The listing builds one solid part. Answer for the finished solid, in the listing's coordinates (mm). Face numbers are marked on the shaded views. Round coordinates to 2 decimals unless told otherwise and drop trailing zeros. Write each loop counter-clockwise with the first axis right and the second up, starting at its lowest first coordinate (ties: lowest second). Pieces come first, ordered by that corner, then holes. Notation, with made-up numbers: (-20, -2) - (24, -2) arc R8 ccw to (24, 8) - close; hole circle Ø5 at (40, 59.25). An arc over 180 degrees is marked (long way). Return JSON: item names as keys, results as strings. Group by question number.
(1) Find the intervals of material crossed by line 1 along Z through (x, y) = (115, 3); line 2 along Y through (x, z) = (117.5, -21); line 3 along Z through (x, y) = (40, 34.5), in increasing order. Write a range as [from, to].
(2) Section A-A, the plane x = 120.5 is taken. Write down the section's boundary in (y, z), then the cut area to 3 significant figures.
(3) Section B-B, the plane x = 165 is taken. Write down the section's boundary in (y, z), then the cut area to 3 significant figures.
(4) Determine the mould class of the marked faces 1, 2, 3 and 4 for opening direction Y: +Y half, -Y half, draft (parallel to the pull), parting line (faces both ways), or undercut.
(5) Each of these flat-tipped pins is pushed along its axis until it touches: pin 1 (8 mm diameter, centred on x = 156, z = -41.5, fed in from +Y); pin 2 (2.5 mm diameter, centred on y = -3, z = 50, fed in from -X); pin 3 (5.5 mm diameter, centred on x = 137.5, y = 35, fed in from -Z); pin 4 (12 mm diameter, centred on y = 22, z = 24.5, fed in from +X). Where does it stop, or does it pass through?
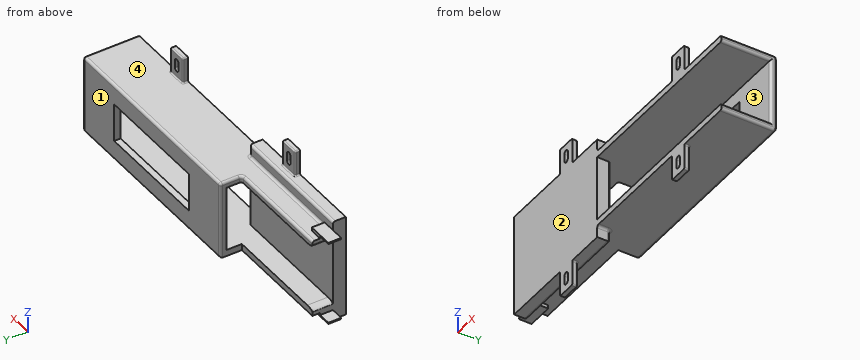
```python
from build123d import *

# Parameters (mm, degrees)
SKETCH1_W                 = 100
SKETCH1_H                 = 80
BOSS_EXTRUDE1_DEPTH       = 5
BOSS_EXTRUDE2_DEPTH       = 15
BOSS_EXTRUDE4_DEPTH       = 150
SKETCH9_W                 = 85
SKETCH9_H                 = 5
BOSS_EXTRUDE5_DEPTH       = 16
SKETCH3_W                 = 15
SKETCH3_H                 = 20
BOSS_EXTRUDE3_DEPTH       = 4
F_4_0MM_START             = -5
F_4_0MM_DOWEL_SLOT1_DEPTH = 4
SKETCH12_W                = 2.75
SKETCH12_H                = 10
BOSS_EXTRUDE7_DEPTH       = 10
SKETCH13_W                = 1
SKETCH13_H                = 10
BOSS_EXTRUDE8_DEPTH       = 10
SKETCH14_W                = 90
SKETCH14_H                = 30
CUT_EXTRUDE1_DEPTH        = 214.187710715
FILLET2_R                 = 2
FILLET3_R                 = 1
FILLET4_SIZE              = 2
FILLET4_SIZE_2            = 6


# Read off the part's stored shape, not the designer's step: Ø4.0mm Dowel Slot1
with BuildPart() as part:
    # Sketch1 → Boss-Extrude1 (new, symmetric)
    with BuildSketch(Plane(origin=(0, 0, 0), x_dir=(1, 0, 0), z_dir=(0, 1, 0))):
        Rectangle(SKETCH1_W, SKETCH1_H)
    extrude(amount=BOSS_EXTRUDE1_DEPTH, both=True)

    # Sketch2 → Boss-Extrude2 (add)
    with BuildSketch(Plane(origin=(50, 0, 0), x_dir=(0, 0, -1), z_dir=(1, 0, 0))):
        Polygon((-30.5, 5), (-30.5, 38), (30.5, 38), (30.5, 5), (25.5, 5), (25.5, 33), (-25.5, 33), (-25.5, 5), align=None)
    extrude(amount=-BOSS_EXTRUDE2_DEPTH)

    # Sketch4 → Boss-Extrude4 (add)
    with BuildSketch(Plane(origin=(50, 0, 0), x_dir=(0, 0, -1), z_dir=(1, 0, 0))):
        Polygon((-30.5, 38), (30.5, 38), (30.5, -5), (25.5, -5), (25.5, 33), (-25.5, 33), (-25.5, -5), (-30.5, -5), align=None)
    extrude(amount=BOSS_EXTRUDE4_DEPTH)

    # Sketch9 → Boss-Extrude5 (add)
    with BuildSketch(Plane(origin=(0, 5, 0), x_dir=(1, 0, 0), z_dir=(0, 1, 0))):
        with Locations((-7.5, -28)):
            Rectangle(SKETCH9_W, SKETCH9_H)
        with Locations((-7.5, 28)):
            Rectangle(SKETCH9_W, SKETCH9_H)
    extrude(amount=BOSS_EXTRUDE5_DEPTH)

    # Sketch3 → Boss-Extrude3 (add)
    with BuildSketch(Plane.XZ.offset(5)):
        with Locations((12.5, 50)):
            Rectangle(SKETCH3_W, SKETCH3_H)
        with Locations((147.5, 40.5)):
            Rectangle(SKETCH3_W, SKETCH3_H)
        with Locations((147.5, -40.5)):
            Rectangle(SKETCH3_W, SKETCH3_H)
        with Locations((12.5, -50)):
            Rectangle(SKETCH3_W, SKETCH3_H)
    extrude(amount=-BOSS_EXTRUDE3_DEPTH)

    # Ø4.0mm Dowel Slot1 outline → Ø4.0mm Dowel Slot1 (cut)
    with BuildSketch(Plane(origin=(0, 0, 0), x_dir=(1, 0, 0), z_dir=(0, 1, 0)).offset(F_4_0MM_START)):
        with BuildLine():
            Line((149.5, 37.5), (149.5, 43.5))
            ThreePointArc((149.5, 43.5), (147.5, 45.5), (145.5, 43.5))
            Line((145.5, 43.5), (145.5, 37.5))
            ThreePointArc((145.5, 37.5), (147.5, 35.5), (149.5, 37.5))
        make_face()
        with BuildLine():
            ThreePointArc((149.5, -37.5), (147.5, -35.5), (145.5, -37.5))
            Line((145.5, -37.5), (145.5, -43.5))
            ThreePointArc((145.5, -43.5), (147.5, -45.5), (149.5, -43.5))
            Line((149.5, -43.5), (149.5, -37.5))
        make_face()
        with BuildLine():
            Line((14.5, -53), (14.5, -47))
            ThreePointArc((14.5, -47), (12.5, -45), (10.5, -47))
            Line((10.5, -47), (10.5, -53))
            ThreePointArc((10.5, -53), (12.5, -55), (14.5, -53))
        make_face()
        with BuildLine():
            ThreePointArc((14.5, 53), (12.5, 55), (10.5, 53))
            Line((10.5, 53), (10.5, 47))
            ThreePointArc((10.5, 47), (12.5, 45), (14.5, 47))
            Line((14.5, 47), (14.5, 53))
        make_face()
    extrude(amount=F_4_0MM_DOWEL_SLOT1_DEPTH, mode=Mode.SUBTRACT)

    # Sketch12 → Boss-Extrude7 (add)
    with BuildSketch(Plane.ZY.offset(50)):
        with Locations((-31.875, 10)):
            Rectangle(SKETCH12_W, SKETCH12_H)
        with Locations((31.875, 10)):
            Rectangle(SKETCH12_W, SKETCH12_H)
    extrude(amount=-BOSS_EXTRUDE7_DEPTH)

    # Sketch13 → Boss-Extrude8 (add)
    with BuildSketch(Plane.ZY.offset(50)):
        with Locations((32.75, 10)):
            Rectangle(SKETCH13_W, SKETCH13_H)
        with Locations((-32.75, 10)):
            Rectangle(SKETCH13_W, SKETCH13_H)
    extrude(amount=BOSS_EXTRUDE8_DEPTH)

    # Sketch14 → Cut-Extrude1 (cut, through all)
    with BuildSketch(Plane(origin=(0, 38, 0), x_dir=(1, 0, 0), z_dir=(0, 1, 0))):
        with Locations((117.5, 0)):
            Rectangle(SKETCH14_W, SKETCH14_H)
    extrude(amount=-CUT_EXTRUDE1_DEPTH, mode=Mode.SUBTRACT)

    # Fillet2
    fillet2_edges = [part.edges().sort_by_distance(p)[0] for p in [
        (0, 5, 40),
        (50, 5, -35.25),
        (5, 5, -30.5),
        (5, 5, 30.5),
        (35, 29.5, 30.5),
        (35, 38, 0),
        (117.5, 38, 30.5),
        (117.5, 38, -30.5),
        (50, 0, 30.5),
        (50, 0, -30.5),
        (50, 5, 35.25),
        (200, 16.5, 30.5),
        (200, 14, 25.5),
        (200, 33, 0),
        (200, 14, -25.5),
        (200, 16.5, -30.5),
        (200, 38, 0),
        (35, 21, 28),
        (-7.5, 21, 30.5),
        (0, 5, -40),
    ]]
    fillet(fillet2_edges, radius=FILLET2_R)

    # Fillet3
    fillet3_edges = [part.edges().sort_by_distance(p)[0] for p in [
        (20, -1, 50),
        (20, -3, 60),
        (12.5, -1, 40),
        (20, -3, 40),
        (5, -1, 50),
        (5, -3, 40),
        (12.5, -1, 60),
        (5, -3, 60),
        (140, -1, 40.5),
        (140, -3, 30.5),
        (147.5, -1, 50.5),
        (140, -3, 50.5),
        (155, -1, 40.5),
        (155, -3, 50.5),
        (147.5, -1, 30.5),
        (155, -3, 30.5),
        (147.5, -1, -30.5),
        (140, -3, -30.5),
        (155, -1, -40.5),
        (155, -3, -30.5),
        (147.5, -1, -50.5),
        (155, -3, -50.5),
        (140, -1, -40.5),
        (140, -3, -50.5),
        (12.5, -1, -40),
        (5, -3, -40),
        (20, -1, -50),
        (20, -3, -40),
        (12.5, -1, -60),
        (20, -3, -60),
        (5, -1, -50),
        (5, -3, -60),
        (50, 5, 0),
    ]]
    fillet(fillet3_edges, radius=FILLET3_R)

    # Fillet4
    # an asymmetric fillet: 6, 2 mm, written as the material it takes off along each edge
    with BuildSketch(Plane(origin=(-50, 5, 25.5), x_dir=(0, 0, 1), z_dir=(0, 1, 0))) as fillet4_piece_1:
        with BuildLine():
            Bezier((FILLET4_SIZE, 0), (0, 0), (0, FILLET4_SIZE_2), weights=[1, 0.707106781, 1])
            Line((0, FILLET4_SIZE_2), (0, 0))
            Line((0, 0), (FILLET4_SIZE, 0))
        make_face()
    extrude(amount=31, mode=Mode.SUBTRACT)
    with BuildSketch(Plane(origin=(-50, 5, -25.5), x_dir=(0, 0, -1), z_dir=(0, 1, 0))) as fillet4_piece_2:
        with BuildLine():
            Bezier((FILLET4_SIZE, 0), (0, 0), (0, -FILLET4_SIZE_2), weights=[1, 0.707106781, 1])
            Line((0, -FILLET4_SIZE_2), (0, 0))
            Line((0, 0), (FILLET4_SIZE, 0))
        make_face()
    extrude(amount=31, mode=Mode.SUBTRACT)


solid = part.part
```
Working result:
{
 "1": {"line 1": "z = [-30.5, -25.5], [25.5, 30.5]", "line 2": "y = [33, 38]", "line 3": "z = [-30.5, 30.5]"},
 "2": {"outline": "(-5, -30.5) - (36, -30.5) arc R2 ccw to (38, -28.5) - (38, -15) - (33, -15) - (33, -25.5) - (-5, -25.5) - close; (-5, 25.5) - (33, 25.5) - (33, 15) - (38, 15) - (38, 28.5) arc R2 ccw to (36, 30.5) - (-5, 30.5) - close", "area": "533 mm^2"},
 "3": {"outline": "(-5, -30.5) - (36, -30.5) arc R2 ccw to (38, -28.5) - (38, 28.5) arc R2 ccw to (36, 30.5) - (-5, 30.5) - (-5, 25.5) - (33, 25.5) - (33, -25.5) - (-5, -25.5) - close", "area": "683 mm^2"},
 "4": {"face 1": "+Y half", "face 2": "-Y half", "face 3": "undercut", "face 4": "draft"},
 "5": {"pin 1": "stops at y = -1", "pin 2": "stops at x = 5", "pin 3": "stops at z = -30.5", "pin 4": "stops at x = 200"}
}
